from build123d import *

# Parameters (mm, degrees)
SKETCH_3_R      = 1.55
EXTRUDE_1_DEPTH = 1.6
SKETCH_4_R      = 0.5
EXTRUDE_2_DEPTH = 6
SKETCH_5_R      = 7
EXTRUDE_3_DEPTH = 4
SKETCH_6_R      = 3.5
EXTRUDE_4_DEPTH = 1.4
SKETCH_7_R      = 5
EXTRUDE_5_DEPTH = 4


with BuildPart() as part:
    # 草图3 → 凸台-拉伸1 (new body)
    with BuildSketch(Plane.XY):
        with BuildLine():
            Line((-6.5, -14), (6.5, -14))
            ThreePointArc((6.5, -14), (12.51040764, -11.51040764), (15, -5.5))
            Line((15, -5.5), (15, 9))
            ThreePointArc((15, 9), (13.535533906, 12.535533906), (10, 14))
            Line((10, 14), (-10, 14))
            ThreePointArc((-10, 14), (-13.535533906, 12.535533906), (-15, 9))
            Line((-15, 9), (-15, -5.5))
            ThreePointArc((-15, -5.5), (-12.51040764, -11.51040764), (-6.5, -14))
        make_face()
        with Locations((12.5, 8.5)):
            Circle(SKETCH_3_R, mode=Mode.SUBTRACT)
        with Locations((12.5, -2.5)):
            Circle(SKETCH_3_R, mode=Mode.SUBTRACT)
        with Locations(Location((-12.5, -2.5, 0), (0, 0, 180))):
            Circle(SKETCH_3_R, mode=Mode.SUBTRACT)
        with Locations(Location((-12.5, 8.5, 0), (0, 0, 180))):
            Circle(SKETCH_3_R, mode=Mode.SUBTRACT)
    extrude(amount=EXTRUDE_1_DEPTH)

    # 草图4 → 凸台-拉伸2 (add)
    with BuildSketch(Plane.XY.offset(1.6)):
        with BuildLine():
            Line((-10.4, 9.4), (-6.9, 12.9))
            Line((-6.9, 12.9), (6.9, 12.9))
            Line((6.9, 12.9), (10.4, 9.4))
            Line((10.4, 9.4), (10.4, 4.5))
            Line((10.4, 4.5), (10.9, 4.5))
            ThreePointArc((10.9, 4.5), (12.9, 2.5), (10.9, 0.5))
            Line((10.9, 0.5), (10.4, 0.5))
            Line((10.4, 0.5), (10.4, -4.4))
            Line((10.4, -4.4), (6.9, -7.9))
            Line((6.9, -7.9), (-6.9, -7.9))
            Line((-6.9, -7.9), (-10.4, -4.4))
            Line((-10.4, -4.4), (-10.4, 0.5))
            Line((-10.4, 0.5), (-10.9, 0.5))
            ThreePointArc((-10.9, 0.5), (-12.9, 2.5), (-10.9, 4.5))
            Line((-10.9, 4.5), (-10.4, 4.5))
            Line((-10.4, 4.5), (-10.4, 9.4))
        make_face()
        with Locations((10.9, 2.5)):
            Circle(SKETCH_4_R, mode=Mode.SUBTRACT)
        with Locations((-10.9, 2.5)):
            Circle(SKETCH_4_R, mode=Mode.SUBTRACT)
    extrude(amount=EXTRUDE_2_DEPTH)

    # 草图5 → 凸台-拉伸3 (add)
    with BuildSketch(Plane.XY.offset(7.6)):
        with Locations((0, 2.5)):
            Circle(SKETCH_5_R)
    extrude(amount=EXTRUDE_3_DEPTH)

    # 草图6 → 凸台-拉伸4 (add)
    with BuildSketch(Plane.XY.offset(11.6)):
        with Locations((0, 2.5)):
            Circle(SKETCH_6_R)
    extrude(amount=EXTRUDE_4_DEPTH)

    # 草图7 → 凸台-拉伸5 (add)
    with BuildSketch(Plane.XY.offset(13)):
        with Locations((0, 2.5)):
            Circle(SKETCH_7_R)
    extrude(amount=EXTRUDE_5_DEPTH)

    # 草图8 → 旋转1 (revolve)
    with BuildSketch(Plane(origin=(0, 2.5, 0), x_dir=(1, 0, 0), z_dir=(0, 1, 0))):
        with BuildLine():
            Line((0, -17), (-4.358898944, -17))
            ThreePointArc((-4.358898944, -17), (-2.236067977, -17.746794345), (0, -18))
            Line((0, -18), (0, -17))
        make_face()
    revolve(axis=Axis((0, 2.5, 17), (0, 0, 1)))


solid = part.part
Can you work these out from the model? Positions are in its coordinate system, mm. A direction names the side the tool comes from. Give positions to 0.01 mm unless a question says otherwise; leave off trailing zeros. Loops run counter-clockwise (first coordinate to the right, second up) from the corner with the lowest first, then second, coordinate; pieces in that order, holes last. Notation, with made-up numbers: M 30.5,-26.75 L 80.5,-26.75 A22 ccw 80.5,-12.75 Z; hole C 30.25,-7 d3. An arc over 180 degrees is marked long. One line per item, written item: value. Start each with the question number.
1) If I drill on line 1 (Y direction, x = 10.9, z = 2.9); line 2 (Y direction, x = 12.5, z = 0.85); line 3 (Z direction, x = -9, y = -6), over which ranges is the centre line in solid material (lowest first)? Write a range as [from, to].
2) On a 3-axis mill with a long thin cutter (end or side, diameter ignored), from which of +Z, -Z, +X, -X, +Y, -Y can I reach the whole of each face in a straight line? I mean faces 5 (the face through (-2, 6, 11.6)), 6 (the face through (12.9, 2.5, 4.6)), 7 (the face through (-8.7, 11.1, 4.6)), 8 (the face through (-8.6, -6.2, 4.6)). Say none if no direction works.
3) I'm going to push flat-ended pins straight in: pin 1 (1.1 mm diameter, centred on x = -11, y = 2.5, fed in from +Z); pin 2 (1 mm diameter, centred on x = -0.5, z = 10.5, fed in from +Y); pin 3 (8 mm diameter, centred on x = 8, z = 15.5, fed in from +Y); pin 4 (8 mm diameter, centred on x = 10, z = 4.5, fed in from +Y). Where does each tip first touch, or does it pass through?
4) If we section it at A-A, the plane z = 2.25: Write out the boundary of the cut face in (x, y), and give its area (3 significant figures).
5) Thinking about a two-plate mould opening in Y: for faces 1 (the face through (-11.27, -1.56, 0.79)), 2 (the face through (0.3, 7, 17)), 3 (the face through (6.677, 4.603, 9.572)), 4 (the face through (11.27, -3.44, 0.79)), which applies, +Y half, -Y half, draft (parallel to the pull), parting line (faces both ways), or undercut?
6) If we section it at D-D, the plane y = -0.25: Write out the boundary of the cut face in (x, z), and give its area (3 significant figures).
7) If we section it at B-B, the plane x = -12.5: Write out the boundary of the cut face in (y, z).
8) If we section it at C-C, the plane x = 0: Write out the boundary of the cut face in (y, z), and give its area (3 significant figures).
Completed:
1. line 1: y = [0.5, 2], [3, 4.5]
1. line 2: y = [-11.52, -4.05], [-0.95, 6.95], [10.05, 13.33]
1. line 3: z = [0, 1.6]
2. face 5: none
2. face 6: +Z, +X
2. face 7: +Z, -X, +Y
2. face 8: +Z, -X, -Y
3. pin 1: stops at z = 7.6
3. pin 2: stops at y = 9.5
3. pin 3: stops at y = 5.5
3. pin 4: stops at y = 14
4. outline: M -10.9,0.5 L -10.4,0.5 L -10.4,-4.4 L -6.9,-7.9 L 6.9,-7.9 L 10.4,-4.4 L 10.4,0.5 L 10.9,0.5 A2 ccw 10.9,4.5 L 10.4,4.5 L 10.4,9.4 L 6.9,12.9 L -6.9,12.9 L -10.4,9.4 L -10.4,4.5 L -10.9,4.5 A2 ccw Z; hole C -10.9,2.5 d1; hole C 10.9,2.5 d1
4. area: 423 mm^2
5. face 1: undercut
5. face 2: draft
5. face 3: parting line
5. face 4: undercut
6. outline: M -15,0 L 15,0 L 15,1.6 L 10.4,1.6 L 10.4,7.6 L 6.44,7.6 L 6.44,11.6 L 2.17,11.6 L 2.17,13 L 4.18,13 L 4.18,17 L 3.38,17 A9.61 ccw -3.38,17 L -4.18,17 L -4.18,13 L -2.17,13 L -2.17,11.6 L -6.44,11.6 L -6.44,7.6 L -10.4,7.6 L -10.4,1.6 L -15,1.6 Z
6. area: 267 mm^2
7. outline: M -11.52,0 L -4.05,0 L -4.05,1.6 L -11.52,1.6 Z; M -0.95,0 L 6.95,0 L 6.95,1.6 L 3.7,1.6 L 3.7,7.6 L 1.3,7.6 L 1.3,1.6 L -0.95,1.6 Z; M 10.05,0 L 13.33,0 L 13.33,1.6 L 10.05,1.6 Z
8. outline: M -14,0 L 14,0 L 14,1.6 L 12.9,1.6 L 12.9,7.6 L 9.5,7.6 L 9.5,11.6 L 6,11.6 L 6,13 L 7.5,13 L 7.5,17 L 6.86,17 A10 ccw -1.86,17 L -2.5,17 L -2.5,13 L -1,13 L -1,11.6 L -4.5,11.6 L -4.5,7.6 L -7.9,7.6 L -7.9,1.6 L -14,1.6 Z
8. area: 281 mm^2
